```python
from build123d import *

# Parameters (mm, degrees)
BOSS_EXTRUDE1_DEPTH      = 3.25
BOSS_EXTRUDE1_DEPTH_BACK = 3.25
SKETCH1_W                = 10
SKETCH1_H                = 0.5
SKETCH1_W_2              = 28
SKETCH1_H_2              = 16
SKETCH1_R                = 1.75
BOSS_EXTRUDE2_DEPTH      = 1.5
BOSS_EXTRUDE2_DEPTH_BACK = 8
SKETCH2_W                = 28
SKETCH2_H                = 16
SKETCH2_R                = 1.75
CUT_EXTRUDE1_DEPTH       = 9.5
CUT_EXTRUDE2_DEPTH       = 1.5
FILLET1_R                = 1
FILLET2_R                = 1
FILLET3_R                = 3
SKETCH5_W                = 3
SKETCH5_H                = 2
BOSS_EXTRUDE3_DEPTH      = 2
FILLET4_R                = 1.5
CUT_EXTRUDE3_DEPTH       = 35.003713088
CUT_EXTRUDE3_DEPTH_BACK  = 2
SKETCH6_W                = 1
SKETCH6_H                = 4


with BuildPart() as part:
    # Sketch1 → Boss-Extrude1 (new, two sides: drawn at the far end of the back side and taken through both)
    # profile 1 of 4: a face of its own
    with BuildSketch(Plane.XY.offset(-BOSS_EXTRUDE1_DEPTH_BACK)):
        with Locations((-5, 6.25)):
            Rectangle(SKETCH1_W, SKETCH1_H)
    # profile 2 of 4: a face of its own
    with BuildSketch(Plane.XY.offset(-BOSS_EXTRUDE1_DEPTH_BACK)):
        with Locations((-5, 11.75)):
            Rectangle(SKETCH1_W, SKETCH1_H)
    # profile 3 of 4: a face of its own
    with BuildSketch(Plane.XY.offset(-BOSS_EXTRUDE1_DEPTH_BACK)):
        with Locations((14, 8)):
            Rectangle(SKETCH1_W_2, SKETCH1_H_2)
        with Locations((2.75, 3.25)):
            Circle(SKETCH1_R, mode=Mode.SUBTRACT)
        with Locations((25.25, 13.25)):
            Circle(SKETCH1_R, mode=Mode.SUBTRACT)
    # profile 4 of 4: a face of its own
    with BuildSketch(Plane.XY.offset(-BOSS_EXTRUDE1_DEPTH_BACK)):
        with BuildLine():
            Line((13, 16), (13.7, 16))
            Line((13.7, 16), (13.7, 18.2))
            ThreePointArc((13.7, 18.2), (13.553553391, 18.553553391), (13.2, 18.7))
            Line((13.2, 18.7), (4, 18.7))
            Line((4, 18.7), (4, 18))
            Line((4, 18), (12.5, 18))
            ThreePointArc((12.5, 18), (12.853553391, 17.853553391), (13, 17.5))
            Line((13, 17.5), (13, 16))
        make_face()
    extrude(amount=BOSS_EXTRUDE1_DEPTH + BOSS_EXTRUDE1_DEPTH_BACK)

    # Sketch2 → Boss-Extrude2 (add, two sides: drawn at the far end of the back side and taken through both)
    with BuildSketch(Plane(origin=(0, 0, -3.25), x_dir=(-1, 0, 0), z_dir=(0, 0, -1)).offset(-BOSS_EXTRUDE2_DEPTH_BACK)):
        with Locations((-14, 8)):
            Rectangle(SKETCH2_W, SKETCH2_H)
        with Locations(Location((-25.25, 13.25, 0), (0, 0, 180))):
            Circle(SKETCH2_R, mode=Mode.SUBTRACT)
        with Locations(Location((-2.75, 3.25, 0), (0, 0, 180))):
            Circle(SKETCH2_R, mode=Mode.SUBTRACT)
    extrude(amount=BOSS_EXTRUDE2_DEPTH + BOSS_EXTRUDE2_DEPTH_BACK)

    # Sketch3 → Cut-Extrude1 (cut)
    with BuildSketch(Plane(origin=(0, 12, 0), x_dir=(1, 0, 0), z_dir=(0, 1, 0))):
        with BuildLine():
            ThreePointArc((-5.25, -1.25), (-4, 0), (-5.25, 1.25))
            add(Edge.make_bspline(
                [(-5.25, 1.25), (-8.75, 0), (-5.25, -1.25)],
                knots=[0.849927106, 0.849927106, 0.849927106, 1.849927106, 1.849927106, 1.849927106], degree=2))
        make_face()
    extrude(amount=-CUT_EXTRUDE1_DEPTH, mode=Mode.SUBTRACT)

    # Sketch4 → Cut-Extrude2 (cut)
    with BuildSketch(Plane(origin=(0, 18.7, 0), x_dir=(1, 0, 0), z_dir=(0, 1, 0))):
        with BuildLine():
            ThreePointArc((8.45, -1.25), (9.7, 0), (8.45, 1.25))
            add(Edge.make_bspline(
                [(8.45, 1.25), (4.95, 0), (8.45, -1.25)],
                knots=[0.849927106, 0.849927106, 0.849927106, 1.849927106, 1.849927106, 1.849927106], degree=2))
        make_face()
    extrude(amount=-CUT_EXTRUDE2_DEPTH, mode=Mode.SUBTRACT)

    # Fillet1
    fillet1_edges = [part.edges().sort_by_distance(p)[0] for p in [
        (-5.25, 6.25, 1.25),
        (-5.25, 6.25, -1.25),
        (-5.25, 11.75, 1.25),
        (-5.25, 11.75, -1.25),
        (8.45, 18.35, -1.25),
        (8.45, 18.35, 1.25),
    ]]
    fillet(fillet1_edges, radius=FILLET1_R)

    # Fillet2
    fillet2_edges = [part.edges().sort_by_distance(p)[0] for p in [
        (-10, 6.25, -3.25),
        (4, 18.35, -3.25),
        (-10, 6.25, 3.25),
        (-10, 11.75, 3.25),
        (4, 18.35, 3.25),
        (-10, 11.75, -3.25),
    ]]
    fillet(fillet2_edges, radius=FILLET2_R)

    # Fillet3
    fillet3_edges = [part.edges().sort_by_distance(p)[0] for p in [
        (0, 16, 0),
        (28, 16, 0),
        (28, 0, 0),
        (0, 0, 0),
    ]]
    fillet(fillet3_edges, radius=FILLET3_R)

    # Sketch5 → Boss-Extrude3 (add)
    with BuildSketch(Plane.XZ):
        with Locations((20.5, -1)):
            Rectangle(SKETCH5_W, SKETCH5_H)
        with Locations((20.5, 1)):
            Rectangle(SKETCH5_W, SKETCH5_H)
    extrude(amount=BOSS_EXTRUDE3_DEPTH)

    # Fillet4
    fillet4_edges = [part.edges().sort_by_distance(p)[0] for p in [
        (19, -2, 0),
        (22, -2, 0),
    ]]
    fillet(fillet4_edges, radius=FILLET4_R - 0.0001)  # a hair under: the kernel refuses the full size

    # Sketch6 → Cut-Extrude3 (cut, two sides: drawn at the far end of the back side and taken through both)
    with BuildSketch(Plane.XZ.offset(-CUT_EXTRUDE3_DEPTH_BACK)):
        with Locations((9.5, 0)):
            Rectangle(SKETCH6_W, SKETCH6_H)
    extrude(amount=CUT_EXTRUDE3_DEPTH + CUT_EXTRUDE3_DEPTH_BACK, mode=Mode.SUBTRACT)


solid = part.part
```
Work out the finished part from the listing and answer in its coordinate system (mm). A direction names the side the tool comes from. Give positions to 0.01 mm unless a question says otherwise; leave off trailing zeros. Write each loop counter-clockwise with the first axis right and the second up, starting at its lowest first coordinate (ties: lowest second). Pieces come first, ordered by that corner, then holes.
(1) The part is cut by section B-B on z = -4. Write down the section's boundary in (x, y), plus the area to 3 significant figures.
Final values:
outline: (0, 3) arc R3 ccw to (3, 0) - (25, 0) arc R3 ccw to (28, 3) - (28, 13) arc R3 ccw to (25, 16) - (3, 16) arc R3 ccw to (0, 13) - close; hole circle Ø3.5 at (2.75, 3.25); hole circle Ø3.5 at (25.25, 13.25)
area: 421 mm2
(2) Which of the six approach directions +Z, -Z, +X, -X, +Y, -Y give full straight-line access (tool end or side, diameter ignored) to faces 1 (the flat face through (-4, 6, -1)), 2 (the flat face through (20, -1, 2)), 3 (the flat face through (13, 17, 0)), 4 (the flat face through (20, -1, -2))?
Final values:
face 1: +Z, -Z, -X, -Y
face 2: +Z, +X, -X, -Y
face 3: +Z, -Z, -X
face 4: -Z, +X, -X, -Y
(3) Flat-ended cylindrical pins translate along their axes: pin 1 Ø1.6 at (x, y) = (20, -0.5) entering from +Z; pin 2 Ø3.5 at (x, z) = (-5.5, 1) entering from +Y; pin 3 Ø2 at (x, z) = (22.5, 0) entering from -Y; pin 4 Ø0.8 at (x, y) = (11, 18) entering from -Z. Find the tip coordinate at first contact, or state that the pin passes through.
Final values:
pin 1: stops at z = 4.75
pin 2: stops at y = 12
pin 3: stops at y = -1.62
pin 4: stops at z = -3.25
(4) The part is cut by section C-C on y = 4.25. Write down the section's boundary in (x, z).
Final values:
outline: (0, -4.75) - (1.31, -4.75) - (1.31, 4.75) - (0, 4.75) - close; (4.19, -4.75) - (28, -4.75) - (28, 4.75) - (4.19, 4.75) - close
(5) Straight lines are drawn through the part: line 1 (Y direction, x = 7.5, z = -1.75); line 2 (X direction, y = 10.5, z = -2.75); line 3 (Y direction, x = 25.25, z = -0.5). For each, find the intervals that lie inside material, in ascending order.
Final values:
line 1: y = 0 to 16, 18 to 18.7
line 2: x = 0 to 28
line 3: y = 0.01 to 11.5, 15 to 15.99
(6) The mould has two halves that part along Z. Classify faces 5 (the flat face through (9.5, 1, -2)), 6 (the cylindrical face through (19.43, -1.55, -0.03)), 7 (the flat face through (14, 8, 4.75)): pulls with the +Z half, pulls with the -Z half, needs draft (parallel to the pull), parting line crosses it, or undercut.
Final values:
face 5: undercut
face 6: needs draft
face 7: pulls with the +Z half
(7) The part is cut by section A-A on z = 0. Count the separate pieces of the cut face and the enclosed holes in it, plus the area to 3 significant figures.
Final values:
separate pieces: 4
enclosed holes: 2
area: 437 mm2
